```python
from build123d import *

# Parameters (mm, degrees)
STOCK_KEEL_BULB_SUPPORT_1_START     = -3.3274
STOCK_KEEL_BULB_SUPPORT_1_OUTLINE_R = 3.3782
STOCK_KEEL_BULB_SUPPORT_1_DEPTH     = 6.6548
FILLET1_R                           = 6.35


# Read off the part's stored shape, not the designer's step: Stock-Keel_bulb_support-1
with BuildPart() as part:
    # Stock-Keel_bulb_support-1 outline → Stock-Keel_bulb_support-1 (new body)
    with BuildSketch(Plane.XY.offset(STOCK_KEEL_BULB_SUPPORT_1_START)):
        Polygon((-223.965917593, 0), (10.136293283, 0), (17.069926246, 19.05), (-223.965917593, 19.05), align=None)
        with Locations((-198.565917593, 9.525)):
            Circle(STOCK_KEEL_BULB_SUPPORT_1_OUTLINE_R, mode=Mode.SUBTRACT)
        with Locations((-84.265917593, 9.525)):
            Circle(STOCK_KEEL_BULB_SUPPORT_1_OUTLINE_R, mode=Mode.SUBTRACT)
    extrude(amount=STOCK_KEEL_BULB_SUPPORT_1_DEPTH)

    # Fillet1
    fillet1_edges = [part.edges().sort_by_distance(p)[0] for p in [
        (-223.965917593, 19.05, 0),
        (-223.965917593, 0, 0),
    ]]
    fillet(fillet1_edges, radius=FILLET1_R)


solid = part.part
```
Model file for the job. Use its own axes, mm. Coordinates: 2 decimals unless noted, no trailing zeros. Write each loop counter-clockwise with the first axis right and the second up, starting at its lowest first coordinate (ties: lowest second). Pieces come first, ordered by that corner, then holes. Notation, with made-up numbers: (43, 5.5) - (87, 5.5) arc R18 ccw to (87, 24.5) - close; hole circle Ø10 at (15.5, -7). An arc over 180 degrees is marked (long way). Use a Markdown table: item, result. Add a question column.
Item 1: Drill centre lines: line 1 along X through (y, z) = (9.5, 2.25); line 2 along X through (y, z) = (7, 0.75); line 3 along X through (y, z) = (1.5, -1). Where is each one in solid material? Low to high.
Item 2: Band-saw the part on A-A, the plane z = 0. Write the cut outline in (x, y) (3 decimals).
Item 3: Drop a flat-ended pin along its axis: pin 1 (6 mm diameter, centred on x = -84.27, y = 9.52, fed in from -Z). Give the stop position or say it passes through.
Item 4: Two-plate mould, pull along X, no slides. Class faces 1 (the face through (-195.344, 10.54, -0.047)), 2 (the face through (-222.155, 17.14, 0.047)), 3 (the face through (13.555, 9.392, -0.047)): pulls with the +X half, pulls with the -X half, needs draft (parallel to the pull), parting line crosses it, or undercut.
Item 5: Band-saw the part on B-B, the plane y = 2.25. Write the cut outline in (x, z), and give its area (3 significant figures).
A:
| question | item | result |
|---|---|---|
| 1 | line 1 | x = -223.97 to -201.94, -195.19 to -87.64, -80.89 to 13.59 |
| 1 | line 2 | x = -223.97 to -200.81, -196.32 to -86.51, -82.02 to 12.68 |
| 1 | line 3 | x = -221.71 to 10.68 |
| 2 | outline | (-223.966, 6.35) arc R6.35 ccw to (-217.616, 0) - (10.136, 0) - (17.07, 19.05) - (-217.616, 19.05) arc R6.35 ccw to (-223.966, 12.7) - close; hole circle Ø6.756 at (-198.566, 9.525); hole circle Ø6.756 at (-84.266, 9.525) |
| 3 | pin 1 | passes through |
| 4 | face 1 | undercut |
| 4 | face 2 | pulls with the -X half |
| 4 | face 3 | pulls with the +X half |
| 5 | outline | (-222.46, -3.33) - (10.96, -3.33) - (10.96, 3.33) - (-222.46, 3.33) - close |
| 5 | area | 1,550 mm² |
